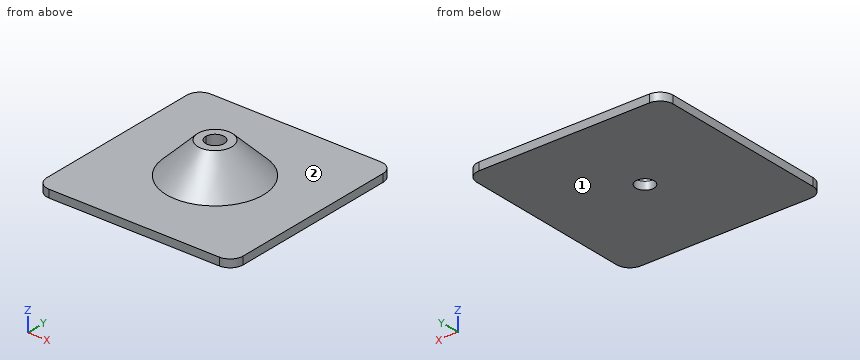
```python
from build123d import *

# Parameters (mm, degrees)
F0_W     = 75
F0_H     = 75
F1_DEPTH = 3
F4_R     = 3.5
F5_DEPTH = 15.001
F6_R     = 5


with BuildPart() as f1:
    # F0 (on Top) → F1 (new body)
    with BuildSketch(Plane.XY):
        Rectangle(F0_W, F0_H)
    extrude(amount=F1_DEPTH)

    # F2 (on Front) → F3 (revolve)
    with BuildSketch(Plane.XZ):
        Polygon((-6.5, 15), (-18.5, 3), (-3.5, 3), (-3.5, 15), align=None)
    revolve(axis=Axis((0, 0, 28.255757), (0, 0, 1)))

    # F4 (on face) → F5 (cut, through all)
    with BuildSketch(Plane.XY.offset(15)):
        Circle(F4_R)
    extrude(amount=-F5_DEPTH, mode=Mode.SUBTRACT)

    # F6
    f6_edges = [f1.edges().sort_by_distance(p)[0] for p in [
        (-37.5, 37.5, 1.5),
        (-37.5, -37.5, 1.5),
        (37.5, -37.5, 1.5),
        (37.5, 37.5, 1.5),
    ]]
    fillet(f6_edges, radius=F6_R)


solid = f1.part
```
Work out the finished part from the listing and answer in its coordinate system (mm). Face numbers are marked on the shaded views. A direction names the side the tool comes from. Round coordinates to 2 decimals unless told otherwise and drop trailing zeros. Loops run counter-clockwise (first coordinate to the right, second up) from the corner with the lowest first, then second, coordinate; pieces in that order, holes last. Notation, with made-up numbers: (44, 77) -> (51, 77) arc R17 ccw to (51, 88) -> close; hole circle Ø2 at (-6.5, 69). An arc over 180 degrees is marked (long way). Write each question's results on one line, items separated by ' | '. Start each with the question number.
1. Given pin 1 Ø8 at (x, z) = (-3.5, 9) entering from -Y; pin 2 Ø2 at (x, y) = (9.5, -9) entering from +Z; pin 3 Ø3 at (y, z) = (18, 6) entering from -X, each flat-ended and moving along its own axis, determine where each tip first touches the part or whether it passes through.
2. Find the intervals of material crossed by probe 1 along Y at (x, z) = (0, 0.6); probe 2 along Z at (x, y) = (4.5, -30), in increasing order. Write a range as from..to.
3. Section D-D (z = 4.25) is taken. Determine the outline of the cut face in (x, y), plus the area to 3 significant figures.
4. Section C-C (x = 25) is taken. Determine the outline of the cut face in (y, z).
5. A tool of negligible diameter and unlimited length cuts with its end or side. For the marked faces 1 and 2, from which of +Z, -Z, +X, -X, +Y, -Y can it reach the whole face along a straight path? Write none if from no direction.
6. Section B-B (z = 8.25) is taken. Determine the outline of the cut face in (x, y).
7. Section A-A (x = 0) is taken. Determine the outline of the cut face in (y, z), plus the area to 3 significant figures.
Evaluation:
1) pin 1: stops at y = -16.2 | pin 2: stops at z = 9.41 | pin 3: passes through
2) probe 1: y = -37.5..-3.5, 3.5..37.5 | probe 2: z = 0..3
3) outline: circle Ø34.5 at (0, 0); hole circle Ø7 at (0, 0) | area: 896 mm2
4) outline: (-37.5, 0) -> (37.5, 0) -> (37.5, 3) -> (-37.5, 3) -> close
5) face 1: -Z, +X, -X, +Y, -Y | face 2: +Z
6) outline: circle Ø26.5 at (0, 0); hole circle Ø7 at (0, 0)
7) outline: (-37.5, 0) -> (-3.5, 0) -> (-3.5, 15) -> (-6.5, 15) -> (-18.5, 3) -> (-37.5, 3) -> close; (3.5, 0) -> (37.5, 0) -> (37.5, 3) -> (18.5, 3) -> (6.5, 15) -> (3.5, 15) -> close | area: 420 mm2
